from build123d import *

# Parameters (mm, degrees)
F0_W        = 40.3080582619
F0_H        = 5.9715644456
F1_DEPTH    = 822
F3_DEPTH    = 196
F5_DEPTH    = 5
F6_T1_DEPTH = 716.1336390313
F8_DEPTH    = 14


# Not quite as in the source:
# - a fillet or chamfer that OpenCascade refuses, or shapes differently, is made with other operations: its cross-section is extruded or revolved along the edge and cut away or added


with BuildPart() as f1:
    # F0 (on Top) → F1 (new body)
    with BuildSketch(Plane.XY):
        Rectangle(F0_W, F0_H)
    extrude(amount=F1_DEPTH)

    # F2 (on Top) → F3 (join)
    with BuildSketch(Plane.XY):
        Polygon((6.5744029718, -8.407556447), (10.5938451005, -1.2962352533), (8.407556447, 6.5744029718), (1.2962352533, 10.5938451005), (-6.5744029718, 8.407556447), (-10.5938451005, 1.2962352533), (-8.407556447, -6.5744029718), (-1.2962352533, -10.5938451005), align=None)
    extrude(amount=-F3_DEPTH)

    # F4 (on Top) → F5 (join)
    with BuildSketch(Plane.XY):
        Polygon((31.1715127681, -0.1368859226), (15.7043030704, 26.9268789703), (-15.4672096977, 27.0637648929), (-31.1715127681, 0.1368859226), (-15.7043030704, -26.9268789703), (15.4672096977, -27.0637648929), align=None)
    extrude(amount=F5_DEPTH)

    # F6: fillet of radius 270.3919189858 on 1 edges, made by hand

    # F6_s2 → F6_t1 (cut)
    with BuildSketch(Plane.XZ.offset(-358.0668195157)):
        with BuildLine():
            ThreePointArc((-20.1540291309, 822), (9.881896476, 753.7882231999), (20.1540291309, 679.9675850829))
            Line((20.1540291309, 679.9675850829), (20.1540291309, 822))
            Line((20.1540291309, 822), (-20.1540291309, 822))
        make_face()
    extrude(amount=F6_T1_DEPTH, mode=Mode.SUBTRACT)

    # F7 (on face) → F8 (join)
    with BuildSketch(Plane(origin=(0, 0, 0), x_dir=(1, 0, 0), z_dir=(0, 0, -1))):
        Polygon((-10.5287277243, 23.8778866657), (-25.9432203033, 2.8207976541), (-15.4144925791, -21.0570890116), (10.5287277243, -23.8778866657), (25.9432203033, -2.8207976541), (15.4144925791, 21.0570890116), align=None)
    extrude(amount=-F8_DEPTH)


solid = f1.part
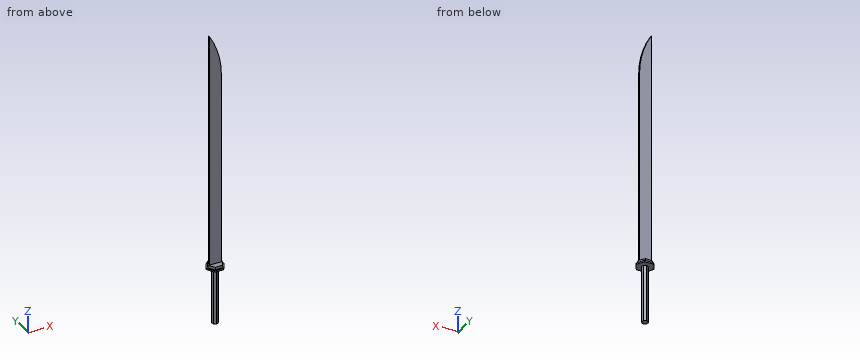
Check sheet for the modelled part. Datum: model origin and axes. Units: mm. Give positions to 0.01 mm unless a question says otherwise; leave off trailing zeros. Write each loop counter-clockwise with the first axis right and the second up, starting at its lowest first coordinate (ties: lowest second). Pieces come first, ordered by that corner, then holes. Notation, with made-up numbers: (80.5, -0.75) -> (113.5, -0.75) arc R32 ccw to (113.5, 27.25) -> close; hole circle Ø10 at (17, 23). An arc over 180 degrees is marked (long way). One line per item, written item: value. Start each with the question number.
Item 1: Material ranges on probe 1 along Y at (x, z) = (16, 501.5); probe 2 along Z at (x, y) = (-24, 10); probe 3 along X at (y, z) = (1.5, 595.5), recorded low to high. Write a range as from..to.
Item 2: Section check B-B on z = 400.5. Record the cut outline in (x, y), then the cut area to 3 significant figures.
Item 3: Section check A-A on z = -133. Record the cut outline in (x, y).
Item 4: Gauge pin test, flat ends, axial feed: pin 1 (6 mm diameter, centred on y = 1.5, z = -45, fed in from -X); pin 2 (3 mm diameter, centred on y = 0.5, z = 267.5, fed in from +X); pin 3 (6.5 mm diameter, centred on y = -1, z = 298.5, fed in from -X). Record the tip position at first contact, or that the pin passes through.
Results list:
1. probe 1: -2.99..2.99
1. probe 2: 0..5
1. probe 3: -20.15..20.15
2. outline: (-20.15, -2.99) -> (20.15, -2.99) -> (20.15, 2.99) -> (-20.15, 2.99) -> close
2. area: 241 mm²
3. outline: (-10.59, 1.3) -> (-8.41, -6.57) -> (-1.3, -10.59) -> (6.57, -8.41) -> (10.59, -1.3) -> (8.41, 6.57) -> (1.3, 10.59) -> (-6.57, 8.41) -> close
4. pin 1: x = -10.59
4. pin 2: x = 20.15
4. pin 3: x = -20.15
